```python
from build123d import *

# Parameters (mm, degrees)
SKETCH1_R           = 75.9206
BOSS_EXTRUDE1_DEPTH = 12.7
SKETCH1_10_R        = 40.4114
CUT_EXTRUDE2_DEPTH  = 13.7
SKETCH2_R           = 12.7
CUT_EXTRUDE3_DEPTH  = 13.7
CUT_EXTRUDE5_DEPTH  = 6.35


with BuildPart() as part:
    # Sketch1 → Boss-Extrude1 (new body)
    with BuildSketch(Plane(origin=(0, 0, 0), x_dir=(1, 0, 0), z_dir=(0, 1, 0))):
        Circle(SKETCH1_R)
    extrude(amount=BOSS_EXTRUDE1_DEPTH)

    # Sketch1<10> → Cut-Extrude2 (cut, through all)
    with BuildSketch(Plane(origin=(0, 0, 0), x_dir=(1, 0, 0), z_dir=(0, 1, 0))):
        Circle(SKETCH1_10_R)
    extrude(amount=CUT_EXTRUDE2_DEPTH, mode=Mode.SUBTRACT)

    # Sketch2 → Cut-Extrude3 (cut, through all)
    with BuildSketch(Plane(origin=(0, 12.7, 0), x_dir=(1, 0, 0), z_dir=(0, 1, 0))):
        with Locations((75.9206, 0)):
            Circle(SKETCH2_R)
    extrude(amount=-CUT_EXTRUDE3_DEPTH, mode=Mode.SUBTRACT)

    # Sketch3 → Cut-Extrude5 (cut)
    with BuildSketch(Plane(origin=(0, 12.7, 0), x_dir=(1, 0, 0), z_dir=(0, 1, 0))):
        Polygon((-28.180043708, 25.701493018), (-25.701493019, 28.180043708), (-60.52670499, 63.00525568), (-63.00525568, 60.52670499), align=None)
        Polygon((28.180043708, 25.701493019), (63.00525568, 60.52670499), (60.52670499, 63.00525568), (25.701493019, 28.180043708), align=None)
        Polygon((25.701493019, -28.180043708), (60.52670499, -63.00525568), (63.00525568, -60.52670499), (28.180043708, -25.701493018), align=None)
        Polygon((-28.180043708, -25.701493019), (-63.00525568, -60.52670499), (-60.52670499, -63.00525568), (-25.701493018, -28.180043708), align=None)
    extrude(amount=-CUT_EXTRUDE5_DEPTH, mode=Mode.SUBTRACT)


solid = part.part
```
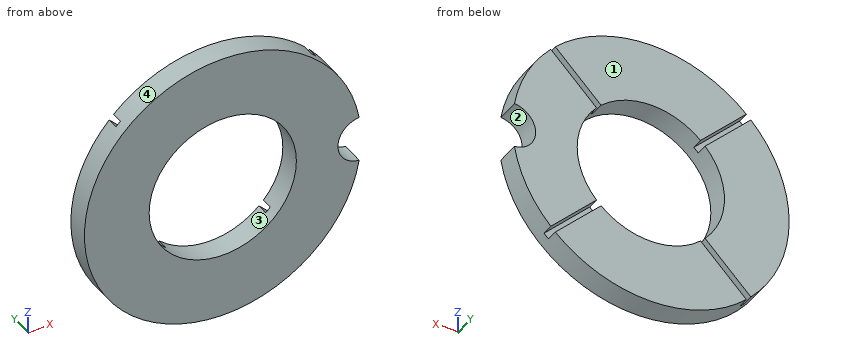
Design review of the part built by this model. Coordinates are the model's own, in mm. Face numbers are marked on the shaded views. Give positions to 0.01 mm unless a question says otherwise; leave off trailing zeros. Write each loop counter-clockwise with the first axis right and the second up, starting at its lowest first coordinate (ties: lowest second). Pieces come first, ordered by that corner, then holes. Notation, with made-up numbers: (63, 12.25) - (85, 12.25) arc R18 cw to (85, 25.25) - close; hole circle Ø5 at (-4.75, 40). An arc over 180 degrees is marked (long way). Return JSON: item names as keys, results as strings. Group by question number.
(1) We need section C-C, the plane z = 0. Give the boundary of the cut face in (x, y).
(2) To check wall thickness, follow probe 1 along X at (y, z) = (7.75, 0); probe 2 along Z at (x, y) = (-1.5, 11); probe 3 along Z at (x, y) = (-30, 10). State the ranges of each line that lie inside material, in increasing order.
(3) Mouldability with a two-part tool opening along X and no side actions: class the marked faces 1, 2, 3 and 4 as +X half, -X half, draft (parallel to the pull), parting line (faces both ways), or undercut.
(4) We need section B-B, the plane x = 0. Give the boundary of the cut face in (y, z), then the cut area to 3 significant figures.
(5) We need section A-A, the plane y = 8.25. Give the boundary of the cut face in (x, z).
(6) We need section D-D, the plane x = -47.5. Give the boundary of the cut face in (y, z), then the cut area to 3 significant figures.
(7) Insertion check: pin 1 (2 mm diameter, centred on y = 7, z = 21.5, fed in from +X); pin 2 (5 mm diameter, centred on x = -37, y = 6.5, fed in from +Z). Each pin has a flat end and moves straight along its axis. Give the tip position at first contact, or say it passes through.
Reported:
{
 "1": {"outline": "(-75.92, 0) - (-40.41, 0) - (-40.41, 12.7) - (-75.92, 12.7) - close; (40.41, 0) - (63.22, 0) - (63.22, 12.7) - (40.41, 12.7) - close"},
 "2": {"probe 1": "x = -75.92 to -40.41, 40.41 to 63.22", "probe 2": "z = -75.91 to -40.38, 40.38 to 75.91", "probe 3": "z = -69.74 to -32.48, -27.52 to -27.08, 27.08 to 27.52, 32.48 to 69.74"},
 "3": {"face 1": "draft", "face 2": "+X half", "face 3": "undercut", "face 4": "parting line"},
 "4": {"outline": "(0, -75.92) - (12.7, -75.92) - (12.7, -40.41) - (0, -40.41) - close; (0, 40.41) - (12.7, 40.41) - (12.7, 75.92) - (0, 75.92) - close", "area": "902 mm2"},
 "5": {"outline": "(-54.91, -52.43) - (-29.79, -27.31) arc R40.41 cw to (-29.79, 27.31) - (-54.91, 52.43) arc R75.92 ccw to start; (-52.43, -54.91) arc R75.92 ccw to (52.43, -54.91) - (27.31, -29.79) arc R40.41 cw to (-27.31, -29.79) - close; (-52.43, 54.91) - (-27.31, 29.79) arc R40.41 cw to (27.31, 29.79) - (52.43, 54.91) arc R75.92 ccw to start; (29.79, -27.31) - (54.91, -52.43) arc R75.92 ccw to (74.86, -12.66) arc R12.7 cw to (74.86, 12.66) arc R75.92 ccw to (54.91, 52.43) - (29.79, 27.31) arc R40.41 cw to start"},
 "6": {"outline": "(0, -59.23) - (12.7, -59.23) - (12.7, -49.98) - (6.35, -49.98) - (6.35, -45.02) - (12.7, -45.02) - (12.7, 45.02) - (6.35, 45.02) - (6.35, 49.98) - (12.7, 49.98) - (12.7, 59.23) - (0, 59.23) - close", "area": "1,440 mm2"},
 "7": {"pin 1": "stops at x = 73.1", "pin 2": "stops at z = 67.63"}
}
